Input: dimensioned drawing with shaded views. Units: mm. Origin: part minimum x, y, z. A direction names the side the tool comes from. Round coordinates to 2 decimals unless told otherwise and drop trailing zeros. Write each loop counter-clockwise with the first axis right and the second up, starting at its lowest first coordinate (ties: lowest second). Pieces come first, ordered by that corner, then holes. Notation, with made-up numbers: M 35,84.5 L 54,84.5 A16 ccw 54,108.5 Z; hole C -15.75,-19 d11. An arc over 180 degrees is marked long. Answer as CSV lines item,"result". Start each with the question number.
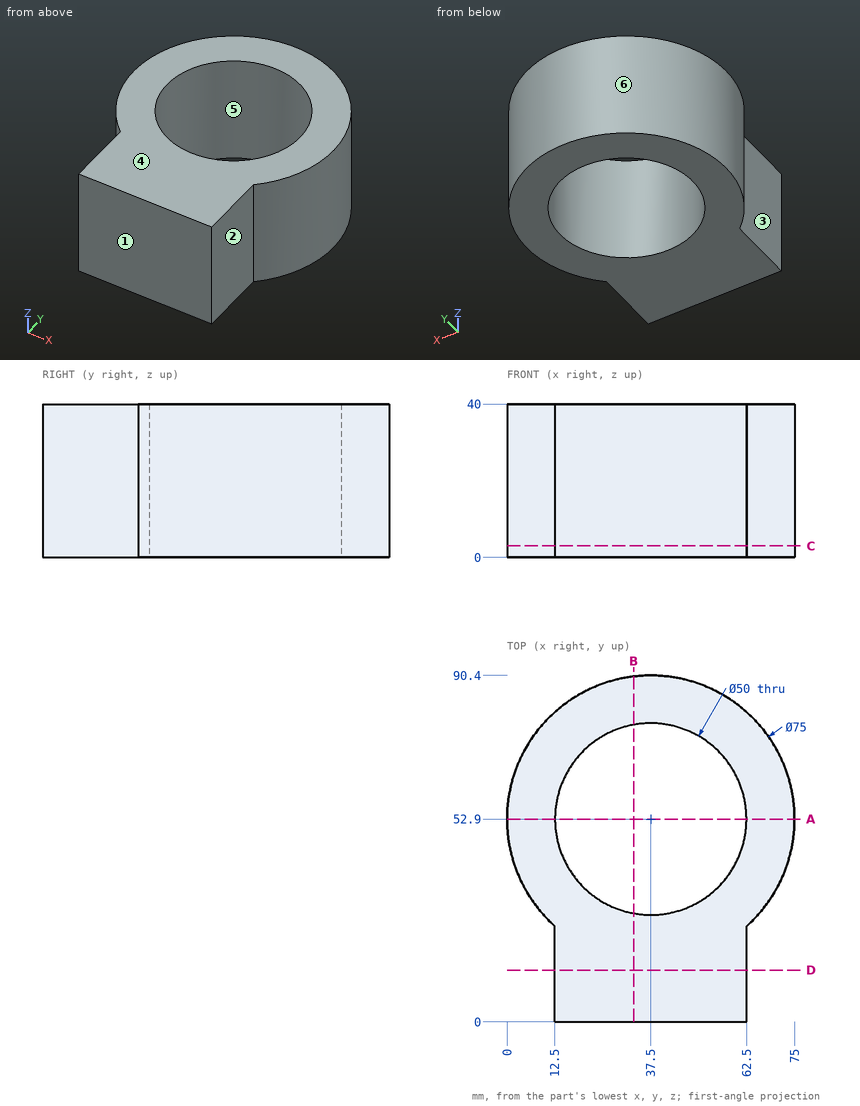
Item 1: Line query: line 1 (Y direction, x = 37, z = 11) (3 decimals); line 2 (Y direction, x = 17, z = 10); line 3 (X direction, y = 61, z = 38.5). Output: solid intervals per line, ascending. Write a range as [from, to].
Item 2: Pin query (flat end, axial travel): pin 1 Ø1.5 at (y, z) = (67, 34) entering from -X; pin 2 Ø4 at (y, z) = (74, 26) entering from +X; pin 3 Ø1 at (y, z) = (25.5, 27) entering from +X; pin 4 Ø1 at (x, y) = (40, 30.5) entering from +Z. Return the tip coordinate at first contact, or that it passes through.
Item 3: Cut plane D-D, the plane y = 13.5. Return loops of the section in (x, z), plus the area to 3 significant figures.
Item 4: Cut plane C-C, the plane z = 3. Return loops of the section in (x, y), plus the area to 3 significant figures.
Item 5: Cut plane B-B, the plane x = 33. Return loops of the section in (y, z).
Item 6: Access query for the marked faces 1, 2 and 3. Directions: +Z, -Z, +X, -X, +Y, -Y. A direction counts if a zero-diameter tool reaches every point of the face in a straight line with its end or side. Return the directions, or none.
Item 7: Cut plane A-A, the plane y = 52.9. Return loops of the section in (x, z), plus the area to 3 significant figures.
Item 8: Draft query along Y for the marked faces 4, 5 and 6. Return one class per face: +Y half, -Y half, draft (parallel to the pull), parting line (faces both ways), or undercut.
Results list:
1,line 1,"[0, 27.905], [77.895, 90.397]"
1,line 2,"[0, 38.59], [67.21, 84.3]"
1,line 3,"[0.89, 13.85], [61.15, 74.11]"
2,pin 1,"x = 2.46"
2,pin 2,"x = 69.77"
2,pin 3,"x = 63.63"
2,pin 4,"through"
3,outline,"M 12.5,0 L 62.5,0 L 62.5,40 L 12.5,40 Z"
3,area,"2,000 mm²"
4,outline,"M 12.5,0 L 62.5,0 L 62.5,24.95 A37.5 ccw long 12.5,24.95 Z; hole C 37.5,52.9 d50"
4,area,"3,370 mm²"
5,outline,"M 0,0 L 28.31,0 L 28.31,40 L 0,40 Z; M 77.49,0 L 90.13,0 L 90.13,40 L 77.49,40 Z"
6,face 1,"+Z, -Z, +X, -X, -Y"
6,face 2,"+Z, -Z, +X, -Y"
6,face 3,"+Z, -Z, -X, -Y"
7,outline,"M 0,0 L 12.5,0 L 12.5,40 L 0,40 Z; M 62.5,0 L 75,0 L 75,40 L 62.5,40 Z"
7,area,"1,000 mm²"
8,face 4,"draft"
8,face 5,"undercut"
8,face 6,"parting line"
